```python
from build123d import *

# Parameters (mm, degrees)
ESBO_O2_R                = 6
RESSALTO_EXTRUS_O1_DEPTH = 324
CHANFRO1_SIZE            = 0.5
ESBO_O3_R                = 6
ESBO_O3_R_2              = 4
CORTE_EXTRUS_O1_DEPTH    = 2.5
ESBO_O4_R                = 6
ESBO_O4_R_2              = 4
CORTE_EXTRUS_O2_DEPTH    = 2.5


with BuildPart() as part:
    # Esboço2 → Ressalto-extrusão1 (new body)
    with BuildSketch(Plane(origin=(0, 0, 0), x_dir=(1, 0, 0), z_dir=(0, 1, 0))):
        with Locations(Location((0, 0, 0), (0, 0, 270))):
            Circle(ESBO_O2_R)
    extrude(amount=RESSALTO_EXTRUS_O1_DEPTH)

    # Chanfro1
    chanfro1_edges = [part.edges().sort_by_distance(p)[0] for p in [
        (0, 0, -6),
        (0, 324, -6),
    ]]
    chamfer(chanfro1_edges, length=CHANFRO1_SIZE)

    # Esboço3 → Corte-extrusão1 (cut, symmetric)
    with BuildSketch(Plane(origin=(0, 5, 0), x_dir=(-1, 0, 0), z_dir=(0, -1, 0))):
        with Locations(Location((0, 0, 0), (0, 0, 90))):
            Circle(ESBO_O3_R)
        with Locations(Location((0, 0, 0), (0, 0, 90))):
            Circle(ESBO_O3_R_2, mode=Mode.SUBTRACT)
    extrude(amount=CORTE_EXTRUS_O1_DEPTH, both=True, mode=Mode.SUBTRACT)

    # Esboço4 → Corte-extrusão2 (cut, symmetric)
    with BuildSketch(Plane(origin=(0, 319, 0), x_dir=(1, 0, 0), z_dir=(0, 1, 0))):
        with Locations(Location((0, 0, 0), (0, 0, 90))):
            Circle(ESBO_O4_R)
        with Locations(Location((0, 0, 0), (0, 0, 90))):
            Circle(ESBO_O4_R_2, mode=Mode.SUBTRACT)
    extrude(amount=CORTE_EXTRUS_O2_DEPTH, both=True, mode=Mode.SUBTRACT)


solid = part.part
```
The model under review builds one solid part; all positions refer to its coordinate system, in mm. A direction names the side the tool comes from. Round coordinates to 2 decimals unless told otherwise and drop trailing zeros. Write each loop counter-clockwise with the first axis right and the second up, starting at its lowest first coordinate (ties: lowest second). Pieces come first, ordered by that corner, then holes. Notation, with made-up numbers: (-1.5, -18) - (22.5, -18) arc R11 ccw to (22.5, -8) - close; hole circle Ø4 at (80.25, 18). An arc over 180 degrees is marked (long way). Use one line per item in the form item = value.
Q1. Tool access review of faces 1 (the cylindrical face through (3.905, 318.965, 0.867)), 2 (the flat face through (0, 324, 0)): name each direction out of +Z, -Z, +X, -X, +Y, -Y from which nothing blocks a thin tool from reaching the whole face with its end or side.
Answer key:
face_1 = none
face_2 = +Z, -Z, +X, -X, +Y
Q2. For line 1 (Y direction, x = 0.25, z = 5); line 2 (Z direction, x = 4.5, y = 49); line 3 (X direction, y = 72, z = -2.25), list the stretches that pass through material, from the lowest coordinate up. Write a range as [from, to].
Answer key:
line_1 = [0, 2.5], [7.5, 316.5], [321.5, 324]
line_2 = [-3.97, 3.97]
line_3 = [-5.56, 5.56]
Q3. Insertion check: pin 1 Ø2 at (y, z) = (110.5, 3) entering from -X; pin 2 Ø5 at (x, z) = (1, -2) entering from -Y; pin 3 Ø5 at (x, y) = (4.5, 81.5) entering from -Z. Each pin has a flat end and moves straight along its axis. Give the tip position at first contact, or say it passes through.
Answer key:
pin_1 = -5.66
pin_2 = 0
pin_3 = -5.66
Q4. Consider section A-A (y = 214). State the section outline as (x, z) points, and give its area (3 significant figures).
Answer key:
outline = circle Ø12 at (0, 0)
area = 113 mm2
Q5. Draft analysis for pull direction Y (two halves, no side actions). For faces 3 (the cylindrical face through (1.802, 159.837, 5.723)), 4 (the flat face through (0, 0, 0)), 5 (the flat face through (-3.92, 7.5, 1.42)), state which applies: +Y half, -Y half, draft (parallel to the pull), parting line (faces both ways), or undercut.
Answer key:
face_3 = draft
face_4 = -Y half
face_5 = undercut
